```python
from build123d import *

# Parameters (mm, degrees)
BOSS_EXTRUDE1_DEPTH = 10
SKETCH2_R           = 8.25
CUT_EXTRUDE1_DEPTH  = 7
CUT_EXTRUDE2_DEPTH  = 16
FILLET2_R           = 3
SKETCH5_R           = 5
CUT_EXTRUDE3_DEPTH  = 16


with BuildPart() as part:
    # Sketch1 → Boss-Extrude1 (new body)
    with BuildSketch(Plane.XY):
        with BuildLine():
            Line((0, 10.25), (100, 10.25))
            ThreePointArc((100, 10.25), (110.25, 0), (100, -10.25))
            Line((100, -10.25), (0, -10.25))
            ThreePointArc((0, -10.25), (-10.25, 0), (0, 10.25))
        make_face()
        with BuildLine():
            Line((92.752155493, -7.247844507), (42.752155493, 42.752155493))
            ThreePointArc((42.752155493, 42.752155493), (42.752155493, 57.247844507), (57.247844507, 57.247844507))
            Line((57.247844507, 57.247844507), (107.247844507, 7.247844507))
            ThreePointArc((107.247844507, 7.247844507), (107.247844507, -7.247844507), (92.752155493, -7.247844507))
        make_face()
        with BuildLine():
            Line((57.247844507, 42.752155493), (7.247844507, -7.247844507))
            ThreePointArc((7.247844507, -7.247844507), (-7.247844507, -7.247844507), (-7.247844507, 7.247844507))
            Line((-7.247844507, 7.247844507), (42.752155493, 57.247844507))
            ThreePointArc((42.752155493, 57.247844507), (57.247844507, 57.247844507), (57.247844507, 42.752155493))
        make_face()
    extrude(amount=BOSS_EXTRUDE1_DEPTH)

    # Sketch2 → Cut-Extrude1 (cut)
    with BuildSketch(Plane.XY.offset(10)):
        with Locations((50, 50)):
            Circle(SKETCH2_R)
        with Locations((100, 0)):
            Circle(SKETCH2_R)
        Circle(SKETCH2_R)
    extrude(amount=-CUT_EXTRUDE1_DEPTH, mode=Mode.SUBTRACT)

    # Sketch4 → Cut-Extrude2 (cut)
    with BuildSketch(Plane.XY.offset(10)):
        Polygon((19.91726189, 8.25), (80.08273811, 8.25), (50, 38.33273811), align=None)
    extrude(amount=-CUT_EXTRUDE2_DEPTH, mode=Mode.SUBTRACT)

    # Fillet2
    fillet2_edges = [part.edges().sort_by_distance(p)[0] for p in [
        (19.91726189, 8.25, 5),
        (50, 38.33273811, 5),
        (80.08273811, 8.25, 5),
    ]]
    fillet(fillet2_edges, radius=FILLET2_R)

    # Sketch5 → Cut-Extrude3 (cut)
    with BuildSketch(Plane.XY.offset(10)):
        Circle(SKETCH5_R)
        with Locations((50, 50)):
            Circle(SKETCH5_R)
        with Locations((100, 0)):
            Circle(SKETCH5_R)
    extrude(amount=-CUT_EXTRUDE3_DEPTH, mode=Mode.SUBTRACT)


solid = part.part
```
The model under review builds one solid part; all positions refer to its coordinate system, in mm. A direction names the side the tool comes from. Coordinates: 2 decimals unless noted, no trailing zeros. Write each loop counter-clockwise with the first axis right and the second up, starting at its lowest first coordinate (ties: lowest second). Pieces come first, ordered by that corner, then holes. Notation, with made-up numbers: (-28, 3.5) - (-14, 3.5) arc R19 cw to (-14, 25.5) - close; hole circle Ø2 at (76, -8). An arc over 180 degrees is marked (long way). Write item = value, one per line.
(1) Consider section C-C, the plane z = 4.75. Give the boundary of the cut face in (x, y), then the cut area to 3 significant figures.
Result sheet:
outline = (-7.25, 7.25) arc R10.25 ccw to (0, -10.25) - (100, -10.25) arc R10.25 ccw to (107.25, 7.25) - (57.25, 57.25) arc R10.25 ccw to (42.75, 57.25) - close; hole circle Ø16.5 at (0, 0); hole (25.04, 13.37) arc R3 ccw to (27.16, 8.25) - (72.84, 8.25) arc R3 ccw to (74.96, 13.37) - (52.12, 36.21) arc R3 ccw to (47.88, 36.21) - close; hole circle Ø16.5 at (50, 50); hole circle Ø16.5 at (100, 0)
area = 3,780 mm^2
(2) Mouldability with a two-part tool opening along X and no side actions: class faces 4 (the face through (104.619, -1.915, 1.521)), 5 (the face through (81.898, 32.598, 4.93)), 6 (the face through (17.402, 31.898, 4.93)), 7 (the face through (51, 2, 0)) as pulls with the +X half, pulls with the -X half, needs draft (parallel to the pull), parting line crosses it, or undercut.
Result sheet:
face_4 = undercut
face_5 = pulls with the +X half
face_6 = pulls with the -X half
face_7 = needs draft
(3) For P1, Ø1, axis at x = 39, z = 5, coming from the +Y side; P2, Ø8, axis at x = 98, y = -1, coming from the +Z side; P3, Ø1.5, axis at y = 6.5, z = 4, coming from the -X side, all flat-tipped, find the tip position at first contact; note any pin that passes through.
Result sheet:
P1 = 54
P2 = 3
P3 = -8.49
(4) Consider section B-B, the plane y = 0. Give the boundary of the cut face in (x, z).
Result sheet:
outline = (-10.25, 0) - (-5, 0) - (-5, 3) - (-8.25, 3) - (-8.25, 10) - (-10.25, 10) - close; (5, 0) - (95, 0) - (95, 3) - (91.75, 3) - (91.75, 10) - (8.25, 10) - (8.25, 3) - (5, 3) - close; (105, 0) - (110.25, 0) - (110.25, 10) - (108.25, 10) - (108.25, 3) - (105, 3) - close
(5) Consider section A-A, the plane x = 50. Give the boundary of the cut face in (y, z).
Result sheet:
outline = (-10.25, 0) - (8.25, 0) - (8.25, 10) - (-10.25, 10) - close; (37.09, 0) - (45, 0) - (45, 3) - (41.75, 3) - (41.75, 10) - (37.09, 10) - close; (55, 0) - (60.25, 0) - (60.25, 10) - (58.25, 10) - (58.25, 3) - (55, 3) - close
(6) Consider section D-D, the plane x = 35.5. Give the boundary of the cut face in (y, z).
Result sheet:
outline = (-10.25, 0) - (8.25, 0) - (8.25, 10) - (-10.25, 10) - close; (23.83, 0) - (50, 0) - (50, 10) - (23.83, 10) - close
(7) Machinability: for faces 1 (the face through (-9.404, -4.078, 4.93)), 2 (the face through (104, -4, 3)), 3 (the face through (75.592, 10.056, 4.93)), which of the approach directions +Z, -Z, +X, -X, +Y, -Y give a long, thin tool a straight path to every point of the face, cutting with its end or side? Answer none if there is none.
Result sheet:
face_1 = +Z, -Z, -X
face_2 = +Z
face_3 = +Z, -Z
(8) For line 1 (X direction, y = 6, z = 9.25); line 2 (Y direction, x = 44, z = 9.25); line 3 (X direction, y = -3, z = 7.75), list the stretches that pass through material, from the lowest coordinate up. Write a range as [from, to].
Result sheet:
line_1 = [-8.31, -5.66], [5.66, 94.34], [105.66, 108.31]
line_2 = [-10.25, 8.25], [32.33, 44.34], [55.66, 58.31]
line_3 = [-9.8, -7.69], [7.69, 92.31], [107.69, 109.8]
